Read the model definition and answer for the solid it produces. Units are mm, in the model's axes. A direction names the side the tool comes from. Give positions to 0.01 mm unless a question says otherwise; leave off trailing zeros. Order: outer loops, then holes, each group sorted by start corner. A loop starts at its lowest first (then second) coordinate and runs counter-clockwise, first axis right, second up. Notation, with made-up numbers: (16, 26) - (53, 26) arc R18 cw to (53, 54) - close; hole circle Ø8 at (-23, 18.5). An arc over 180 degrees is marked (long way). Write each question's results on one line, items separated by ' | '. Start each with the question number.
Q1. Flat-ended cylindrical pins translate along their axes: P1, Ø3, axis at x = 2.5, y = 54, coming from the +Z side; P2, Ø2.5, axis at x = 5, y = 60, coming from the +Z side; P3, Ø4, axis at y = 70.5, z = -4.5, coming from the +X side; P4, Ø1.2, axis at x = 5, z = -3, coming from the -Y side. Find the tip coordinate at first contact, or state that the pin passes through.
Q2. For a pull along Y with two mould halves and no side action, classify faces 5 (the face through (4.93, 9.49, 4.38)), 6 (the face through (2.014, 58.244, -3.26)), 7 (the face through (18, 59, -1)) as +Y half, -Y half, draft (parallel to the pull), parting line (faces both ways), or undercut.
Q3. Find section B-B on x = 5. Count the separate pieces of the cut face and the enclosed holes in it, and give its area (3 significant figures).
Q4. Find section A-A on y = 32.5. Give the vertices of the cut face in (x, z), and give its area (3 significant figures).
Q5. A tool of negligible diameter and unlimited length cuts with its end or side. For faces 1 (the face through (1.986, 61.708, -3.26)), 2 (the face through (10, 21, 2)), 3 (the face through (5, 42, 1)), 4 (the face through (18, 60, -4)), from which of +Z, -Z, +X, -X, +Y, -Y can it reach the whole face along a straight path? Write none if from no direction.
Q6. Find section C-C on y = 73. Give the vertices of the cut face in (x, z), and give its area (3 significant figures).
Q7. Find section D-D on z = 0. Give the vertices of the cut face in (x, y).
Q8. Find the intervals of material crossed by line 1 along Z through (x, y) = (6, 50.5); line 2 along X through (y, z) = (20, 1.7); line 3 along X through (y, z) = (31.5, 3), in increasing order. Write a range as from..to.
from build123d import *

# Parameters (mm, degrees)
SKETCH_R        = 10
PAD_DEPTH       = 10
HOLE_DEPTH      = 0.001
HOLE_FACE4_R    = 5
POCKET_DEPTH    = 11
SKETCH001_W     = 75
SKETCH001_H     = 3
PAD001_DEPTH    = 10
SKETCH002_W     = 5.5
SKETCH002_H     = 2
POCKET001_DEPTH = 10
FILLET_R        = 3
FILLET001_R     = 3
POCKET002_DEPTH = 1.5
SKETCH004_R     = 2
POCKET003_DEPTH = 7
CHAMFER_SIZE    = 2
SKETCH005_R     = 2
POCKET004_DEPTH = 7
CHAMFER001_SIZE = 2
SKETCH006_W     = 28
SKETCH006_H     = 3
PAD002_DEPTH    = 38
FILLET002_R     = 12


with BuildPart() as part:
    # Sketch → Pad (new body)
    with BuildSketch(Plane.YZ):
        Circle(SKETCH_R)
    extrude(amount=PAD_DEPTH)

    # Sketch → Hole (cut, through all)
    with BuildSketch(Plane.YZ):
        Circle(SKETCH_R)
    extrude(amount=-HOLE_DEPTH, mode=Mode.SUBTRACT)

    # Hole Face4 → Pocket (cut)
    with BuildSketch(Plane(origin=(0, 0, 0), x_dir=(0, 1, 0), z_dir=(-1, 0, 0))):
        Circle(HOLE_FACE4_R)
    extrude(amount=-POCKET_DEPTH, mode=Mode.SUBTRACT)

    # Sketch001 → Pad001 (join)
    with BuildSketch(Plane.YZ):
        with Locations((42.5, 2.5)):
            Rectangle(SKETCH001_W, SKETCH001_H)
        with Locations((42.5, -2.5)):
            Rectangle(SKETCH001_W, SKETCH001_H)
    extrude(amount=PAD001_DEPTH)

    # Sketch002 (on Face2 of Pad001) → Pocket001 (cut)
    with BuildSketch(Plane(origin=(0, 0, 0), x_dir=(0, 1, 0), z_dir=(-1, 0, 0))):
        with Locations((7.25, 0)):
            Rectangle(SKETCH002_W, SKETCH002_H)
    extrude(amount=-POCKET001_DEPTH, mode=Mode.SUBTRACT)

    # Fillet
    fillet_edges = [part.edges().sort_by_distance(p)[0] for p in [
        (5, 9.165151, -4),
    ]]
    fillet(fillet_edges, radius=FILLET_R)

    # Fillet001
    fillet001_edges = [part.edges().sort_by_distance(p)[0] for p in [
        (5, 9.165151, 4),
    ]]
    fillet(fillet001_edges, radius=FILLET001_R)

    # Sketch003 (on Face17 of Fillet001) → Pocket002 (cut)
    with BuildSketch(Plane.YX.offset(4)):
        Polygon((23.464102, 3), (23.464102, 7), (20, 9), (16.535898, 7), (16.535898, 3), (20, 1), align=None)
        Polygon((63.464102, 3), (63.464102, 7), (60, 9), (56.535898, 7), (56.535898, 3), (60, 1), align=None)
    extrude(amount=-POCKET002_DEPTH, mode=Mode.SUBTRACT)

    # Sketch004 (on Face13 of Pocket002) → Pocket003 (cut)
    with BuildSketch(Plane(origin=(0, 0, 4), x_dir=(0, -1, 0), z_dir=(0, 0, 1))):
        with Locations((-20, 5)):
            Circle(SKETCH004_R)
    extrude(amount=-POCKET003_DEPTH, mode=Mode.SUBTRACT)

    # Chamfer
    chamfer_edges = [part.edges().sort_by_distance(p)[0] for p in [
        (5, 22, 4),
    ]]
    chamfer(chamfer_edges, length=CHAMFER_SIZE)

    # Sketch005 (on Face40 of Chamfer) → Pocket004 (cut)
    with BuildSketch(Plane.YX.offset(2.5)):
        with Locations((60, 5)):
            Circle(SKETCH005_R)
    extrude(amount=-POCKET004_DEPTH, mode=Mode.SUBTRACT)

    # Chamfer001
    chamfer001_edges = [part.edges().sort_by_distance(p)[0] for p in [
        (5, 58, 4),
    ]]
    chamfer(chamfer001_edges, length=CHAMFER001_SIZE)

    # Sketch006 (on Face6 of Chamfer001) → Pad002 (join)
    with BuildSketch(Plane.YZ.offset(10)):
        with Locations((66, -2.5)):
            Rectangle(SKETCH006_W, SKETCH006_H)
    extrude(amount=PAD002_DEPTH)

    # Fillet002
    fillet002_edges = [part.edges().sort_by_distance(p)[0] for p in [
        (48, 52, -2.5),
        (48, 80, -2.5),
    ]]
    fillet(fillet002_edges, radius=FILLET002_R)


solid = part.part
Working result:
1) P1: z = 4 | P2: through | P3: x = 47.99 | P4: y = -9.71
2) face 5: +Y half | face 6: undercut | face 7: draft
3) separate pieces: 5 | enclosed holes: 0 | area: 584 mm²
4) outline: (0, -4) - (10, -4) - (10, -1) - (0, -1) - close; (0, 1) - (10, 1) - (10, 4) - (0, 4) - close | area: 60.0 mm²
5) face 1: -Z | face 2: +Z, +X, -Y | face 3: +X, -X, +Y | face 4: -Z, +X, -X, +Y
6) outline: (0, -4) - (46.91, -4) - (46.91, -1) - (0, -1) - close; (0, 1) - (10, 1) - (10, 4) - (0, 4) - close | area: 171 mm²
7) outline: (0, -10) - (10, -10) - (10, -5) - (0, -5) - close
8) line 1: -4..-1, 1..4 | line 2: 0..3, 7..10 | line 3: 0..10
